Drawing for the job (mm, zero at the part's lowest x, y, z). A direction names the side the tool comes from. Coordinates: 2 decimals unless noted, no trailing zeros. Order: outer loops, then holes, each group sorted by start corner. A loop starts at its lowest first (then second) coordinate and runs counter-clockwise, first axis right, second up. Notation, with made-up numbers: (86.25, -28) - (145.25, -28) arc R23 ccw to (145.25, -9) - close; hole circle Ø5 at (-40, 81.25). An arc over 180 degrees is marked (long way). Answer as CSV lines item,"result". Start each with the question number.
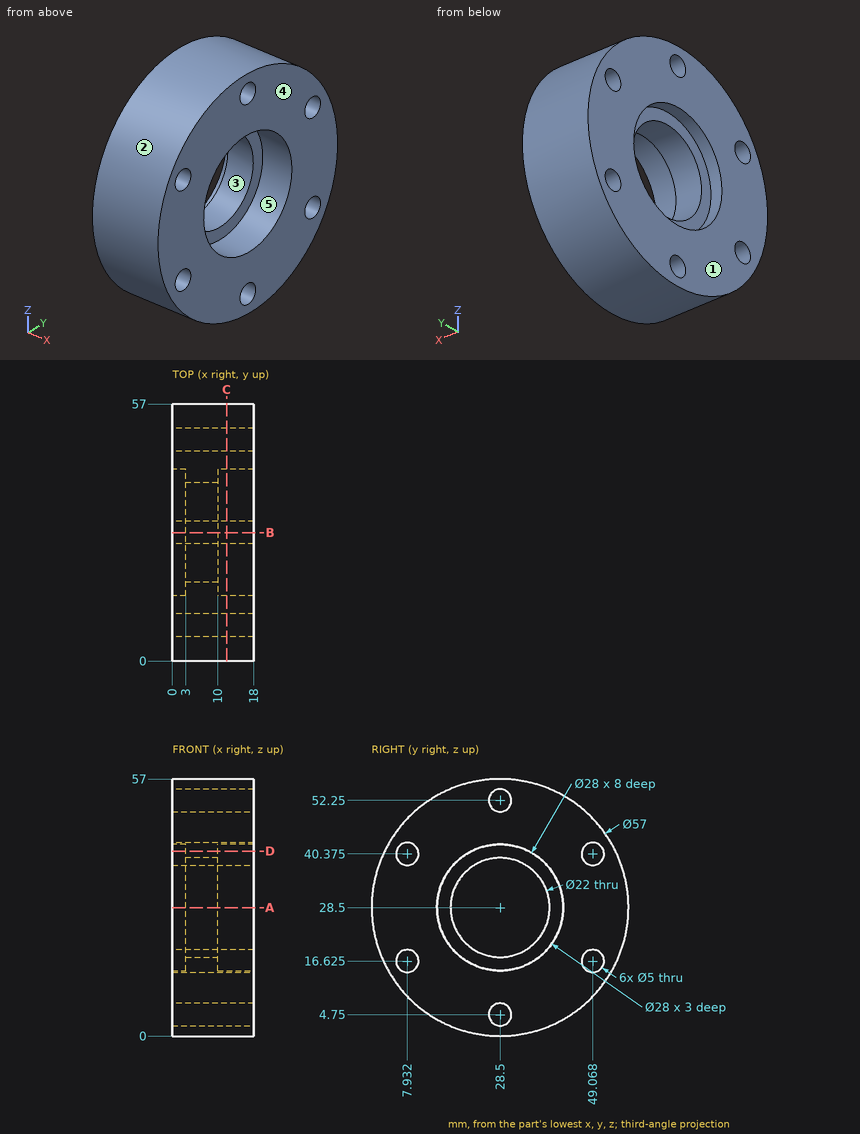
(1) Band-saw the part on A-A on z = 28.5. List the corners of the cut face in (x, y).
(2) Pull direction Z, two halves, no side cores. Call the marked faces 1, 2 and 3: +Z half, -Z half, draft (parallel to the pull), parting line (faces both ways), or undercut.
(3) Which spindle directions (+Z, -Z, +X, -X, +Y, -Y) get a long thin tool onto all of the face, cutting with end or side? Do the marked faces 4 and 5. Say none if no direction does.
(4) Band-saw the part on D-D on z = 41. List the corners of the cut face in (x, y), plus the area to 3 significant figures.
(5) Drop flat-ended pins along their axis: pin 1 Ø6.5 at (y, z) = (49.07, 40.38) entering from +X; pin 2 Ø1.5 at (x, z) = (7, 48) entering from -Y; pin 3 Ø3 at (x, z) = (10.5, 43) entering from -Y; pin 4 Ø4.5 at (y, z) = (49.07, 16.62) entering from -X. Give the stop position or say it passes through.
(6) Band-saw the part on C-C on x = 12. List the corners of the cut face in (y, z) (3 decimals), plus the area to 3 significant figures.
(7) Probe L1, parallel to Y at x = 15.25, z = 38.5 (1 decimal); L2, parallel to Z at x = 14.75, y = 49.5; L3, parallel to Y at x = 16.5, z = 28.5. List the from-to ranges inside material, lowest first. Write a range as [from, to].
(8) Band-saw the part on B-B on y = 28.5. List the corners of the cut face in (x, z).
Filled in:
1,outline,"(0, 0) - (18, 0) - (18, 14.5) - (10, 14.5) - (10, 17.5) - (3, 17.5) - (3, 14.5) - (0, 14.5) - close; (0, 42.5) - (3, 42.5) - (3, 39.5) - (10, 39.5) - (10, 42.5) - (18, 42.5) - (18, 57) - (0, 57) - close"
2,face 1,"draft"
2,face 2,"parting line"
2,face 3,"undercut"
3,face 4,"+Z, -Z, +X, +Y, -Y"
3,face 5,"+X"
4,outline,"(0, 2.89) - (18, 2.89) - (18, 5.51) - (0, 5.51) - close; (0, 10.35) - (18, 10.35) - (18, 22.2) - (10, 22.2) - (10, 34.8) - (18, 34.8) - (18, 46.65) - (0, 46.65) - (0, 34.8) - (3, 34.8) - (3, 22.2) - (0, 22.2) - close; (0, 51.49) - (18, 51.49) - (18, 54.11) - (0, 54.11) - close"
4,area,"609 mm^2"
5,pin 1,"stops at x = 18"
5,pin 2,"stops at y = 7.04"
5,pin 3,"stops at y = 3.14"
5,pin 4,"passes through"
6,outline,"circle Ø57 at (28.5, 28.5); hole circle Ø5 at (7.932, 16.625); hole circle Ø5 at (7.932, 40.375); hole circle Ø28 at (28.5, 28.5); hole circle Ø5 at (28.5, 4.75); hole circle Ø5 at (28.5, 52.25); hole circle Ø5 at (49.068, 16.625); hole circle Ø5 at (49.068, 40.375)"
6,area,"1,820 mm^2"
7,L1,"y = [1.8, 6.3], [9.6, 18.7], [38.3, 47.4], [50.7, 55.2]"
7,L2,"z = [9.23, 14.16], [19.09, 37.91], [42.84, 47.77]"
7,L3,"y = [0, 14.5], [42.5, 57]"
8,outline,"(0, 0) - (18, 0) - (18, 2.25) - (0, 2.25) - close; (0, 7.25) - (18, 7.25) - (18, 14.5) - (10, 14.5) - (10, 17.5) - (3, 17.5) - (3, 14.5) - (0, 14.5) - close; (0, 42.5) - (3, 42.5) - (3, 39.5) - (10, 39.5) - (10, 42.5) - (18, 42.5) - (18, 49.75) - (0, 49.75) - close; (0, 54.75) - (18, 54.75) - (18, 57) - (0, 57) - close"
